For this review, take the finished solid that the model builds, in its own axes (mm). A direction names the side the tool comes from. Round coordinates to 2 decimals unless told otherwise and drop trailing zeros. Write each loop counter-clockwise with the first axis right and the second up, starting at its lowest first coordinate (ties: lowest second). Pieces come first, ordered by that corner, then holes. Notation, with made-up numbers: M 53.25,57.5 L 103.25,57.5 A26 ccw 103.25,72.5 Z; hole C 75.25,38 d6. An arc over 180 degrees is marked long. Answer in a Markdown table with one row per item.
```python
from build123d import *

# Parameters (mm, degrees)
ESQUISSE1_R                         = 9.5
BOSS_EXTRU_1_DEPTH                  = 7
ESQUISSE2_W                         = 5.5
ESQUISSE2_H                         = 2.2
ENL_V_MAT_EXTRU_1_DEPTH             = 6
ENL_V_MAT_EXTRU_2_REACH             = 19.336
ESQUISSE3_R                         = 1.6
ENL_V_MAT_EXTRU_2_DIRECTION_2_REACH = 19.336
ESQUISSE7_R                         = 2.75
ENL_V_MAT_EXTRU_4_DEPTH             = 22.943108417
CHANFREIN2_SIZE                     = 1


with BuildPart() as part:
    # Esquisse1 → Boss.-Extru.1 (new body)
    with BuildSketch(Plane.XY):
        Circle(ESQUISSE1_R)
        with BuildLine():
            Line((-1.565247584, 2.2), (1.565247584, 2.2))
            ThreePointArc((1.565247584, 2.2), (0, -2.7), (-1.565247584, 2.2))
        make_face(mode=Mode.SUBTRACT)
    extrude(amount=BOSS_EXTRU_1_DEPTH)

    # Esquisse2 → Enlèv. mat.-Extru.1 (cut)
    with BuildSketch(Plane(origin=(0, 0, 0), x_dir=(-1, 0, 0), z_dir=(0, 0, -1))):
        with Locations((0, 4.3)):
            Rectangle(ESQUISSE2_W, ESQUISSE2_H)
    extrude(amount=-ENL_V_MAT_EXTRU_1_DEPTH, mode=Mode.SUBTRACT)

    # Esquisse3 → Enlèv. mat.-Extru.2 (cut, up to next)
    with BuildSketch(Plane(origin=(0, 3.2, 0), x_dir=(1, 0, 0), z_dir=(0, 1, 0)), mode=Mode.PRIVATE) as enl_v_mat_extru_2_sk1:
        with Locations(Location((0, -3, 0), (0, 0, 90))):
            Circle(ESQUISSE3_R)
    enl_v_mat_extru_2_tool1 = extrude(enl_v_mat_extru_2_sk1.sketch, amount=-ENL_V_MAT_EXTRU_2_REACH, mode=Mode.PRIVATE) & part.part
    add(enl_v_mat_extru_2_tool1.solids().sort_by_distance((0, 3.2, 3))[0], mode=Mode.SUBTRACT)

    # Esquisse3 → Enlèv. mat.-Extru.2 direction 2 (cut, up to next)
    with BuildSketch(Plane(origin=(0, 3.2, 0), x_dir=(1, 0, 0), z_dir=(0, 1, 0)), mode=Mode.PRIVATE) as enl_v_mat_extru_2_direction_2_sk1:
        with Locations(Location((0, -3, 0), (0, 0, 90))):
            Circle(ESQUISSE3_R)
    enl_v_mat_extru_2_direction_2_tool1 = extrude(enl_v_mat_extru_2_direction_2_sk1.sketch, amount=ENL_V_MAT_EXTRU_2_DIRECTION_2_REACH, mode=Mode.PRIVATE) & part.part
    add(enl_v_mat_extru_2_direction_2_tool1.solids().sort_by_distance((0, 3.2, 3))[0], mode=Mode.SUBTRACT)

    # Esquisse7 → Enlèv. mat.-Extru.4 (cut, through all)
    with BuildSketch(Plane(origin=(0, 9, 0), x_dir=(1, 0, 0), z_dir=(0, 1, 0))):
        with Locations(Location((0, -3, 0), (0, 0, 90))):
            Circle(ESQUISSE7_R)
    extrude(amount=ENL_V_MAT_EXTRU_4_DEPTH, mode=Mode.SUBTRACT)

    # Chanfrein2
    chanfrein2_edges = [part.edges().sort_by_distance(p)[0] for p in [
        (0, 9, 4.6),
    ]]
    chamfer(chanfrein2_edges, length=CHANFREIN2_SIZE)


solid = part.part
```
Q1. Insertion check: P1, Ø1.8, axis at y = 4.5, z = 4.5, coming from the -X side; P2, Ø0.7, axis at x = 0, y = 4, coming from the -Z side; P3, Ø1.6, axis at x = 0.5, z = 1.5, coming from the +Y side. Each pin has a flat end and moves straight along its axis. Give the tip position at first contact, or say it passes through.
Found:
| item | result |
|---|---|
| P1 | x = -8.79 |
| P2 | z = 6 |
| P3 | y = 8.78 |
Q2. Mouldability with a two-part tool opening along Y and no side actions: class faces 1 (the face through (-2.2, -2, 0)), 2 (the face through (-2.059, -9.274, 3.451)), 3 (the face through (0, 2.2, 6)) as +Y half, -Y half, draft (parallel to the pull), parting line (faces both ways), or undercut.
Found:
| item | result |
|---|---|
| face 1 | draft |
| face 2 | parting line |
| face 3 | undercut |
Q3. Take a section at B-B (y = 0). State the section outline as (x, z) points.
Found:
| item | result |
|---|---|
| outline | M -9.5,0 L -2.7,0 L -2.7,7 L -9.5,7 Z; M 2.7,0 L 9.5,0 L 9.5,7 L 2.7,7 Z |
Q4. Take a section at D-D (z = 3). State the section outline as (x, y) points.
Found:
| item | result |
|---|---|
| outline | M -2.75,3.2 L -2.75,5.4 L -1.6,5.4 L -1.6,8 L -2.6,9 L -2.75,9 L -2.75,9.09 A9.5 ccw long 2.75,9.09 L 2.75,9 L 2.6,9 L 1.6,8 L 1.6,5.4 L 2.75,5.4 L 2.75,3.2 L 1.6,3.2 L 1.6,2.17 A2.7 cw long -1.6,2.17 L -1.6,3.2 Z |
Q5. Take a section at C-C (z = 6.5). State the section outline as (x, y) points.
Found:
| item | result |
|---|---|
| outline | C 0,0 d19; hole M -1.57,2.2 A2.7 ccw long 1.57,2.2 Z |
Q6. Machinability: for faces 4 (the face through (0.97, 6.68, 4.27)), 5 (the face through (0, 2.2, 1)), 6 (the face through (-2.75, 4, 3)), which of the approach directions +Z, -Z, +X, -X, +Y, -Y give a long, thin tool a straight path to every point of the face, cutting with its end or side? Answer none if there is none.
Found:
| item | result |
|---|---|
| face 4 | +Y |
| face 5 | +Z, -Z |
| face 6 | -Z |
Q7. For probe 1 along Y at (x, z) = (0, 5.25); probe 2 along X at (y, z) = (0.5, 4.25); probe 3 along Y at (x, z) = (0.75, 5), list the stretches that pass through material, from the lowest coordinate up.
Found:
| item | result |
|---|---|
| probe 1 | -9.5 to -2.7, 2.2 to 3.2, 5.4 to 8.65 |
| probe 2 | -9.49 to -2.65, 2.65 to 9.49 |
| probe 3 | -9.47 to -2.59, 2.2 to 3.2, 5.4 to 8.54 |
Q8. Take a section at A-A (x = 0). State the section outline as (y, z) points, then the cut area to 3 significant figures.
Found:
| item | result |
|---|---|
| outline | M -9.5,0 L -2.7,0 L -2.7,7 L -9.5,7 Z; M 2.2,0 L 3.2,0 L 3.2,1.4 L 2.2,1.4 Z; M 2.2,4.6 L 3.2,4.6 L 3.2,6 L 5.4,6 L 5.4,4.6 L 8,4.6 L 9,5.6 L 9,5.75 L 9.5,5.75 L 9.5,7 L 2.2,7 Z; M 5.4,0 L 9.5,0 L 9.5,0.25 L 9,0.25 L 9,0.4 L 8,1.4 L 5.4,1.4 Z |
| area | 67.0 mm² |
